Could you check a few things on this model? Use its own coordinates, in mm. Coordinates: 2 decimals unless noted, no trailing zeros. Order: outer loops, then holes, each group sorted by start corner. A loop starts at its lowest first (then second) coordinate and runs counter-clockwise, first axis right, second up. Notation, with made-up numbers: (-23, -33) -> (3, -33) arc R18 ccw to (3, -27) -> close; hole circle Ø7 at (23.25, 59.5). An arc over 180 degrees is marked (long way). Use a Markdown table: item, result. Add a question column.
1) If I drill on L1, parallel to Z at x = 15, y = 1.35; L2, parallel to Z at x = 0, y = 1.9; L3, parallel to X at y = 0.7, z = -21, over which ranges is the centre line in solid material (lowest first)? Write a range as [from, to].
2) If we section it at D-D (x = -20): Write out the boundary of the cut face in (y, z).
3) If we section it at B-B (z = 45.5): Write out the boundary of the cut face in (x, y).
4) Will these pins go through, and if not, where does the flat tip stop? pin 1 Ø0.6 at (y, z) = (1, 10.5) entering from +X; pin 2 Ø0.6 at (y, z) = (0.5, 2) entering from +X; pin 3 Ø1 at (y, z) = (0.5, -11) entering from +X; pin 4 Ø1.8 at (x, z) = (20, -34.64) entering from +Y.
5) If we section it at A-A (x = -12): Write out the boundary of the cut face in (y, z), plus the area to 3 significant figures.
6) Thinking about a two-plate mould opening in X: for faces 1 (the flat face through (28.38, 0.99, -41.2)), 2 (the flat face through (8, 2, -1)), 3 (the flat face through (-28.38, 0.99, 41.2)), 4 (the cylindrical face through (-20.45, 0.99, 33.21)), which applies, +X half, -X half, draft (parallel to the pull), parting line (faces both ways), or undercut?
7) If we section it at C-C (z = 15): Write out the boundary of the cut face in (x, y).
```python
from build123d import *

# Parameters (mm, degrees)
SKETCH1_R           = 1.5
BOSS_EXTRUDE1_DEPTH = 2
CUT_EXTRUDE1_DEPTH  = 2


with BuildPart() as part:
    # Sketch1 → Boss-Extrude1 (new body)
    with BuildSketch(Plane(origin=(0, 0, 0), x_dir=(1, 0, 0), z_dir=(0, 1, 0))):
        with BuildLine():
            Line((-31.856435644, 6.435643564), (-25, 75))
            Line((-25, 75), (25, 75))
            Line((25, 75), (31.856435644, 6.435643564))
            ThreePointArc((31.856435644, 6.435643564), (32.5, 0), (31.856435644, -6.435643564))
            Line((31.856435644, -6.435643564), (25, -75))
            Line((25, -75), (-25, -75))
            Line((-25, -75), (-31.856435644, -6.435643564))
            ThreePointArc((-31.856435644, -6.435643564), (-32.5, 0), (-31.856435644, 6.435643564))
        make_face()
        with Locations(Location((-20, 34.641016151, 0), (0, 0, 270))):
            Circle(SKETCH1_R, mode=Mode.SUBTRACT)
        with Locations(Location((20, 34.641016151, 0), (0, 0, 90))):
            Circle(SKETCH1_R, mode=Mode.SUBTRACT)
        with Locations(Location((20, -34.641016151, 0), (0, 0, 270))):
            Circle(SKETCH1_R, mode=Mode.SUBTRACT)
        with Locations(Location((-20, -34.641016151, 0), (0, 0, 90))):
            Circle(SKETCH1_R, mode=Mode.SUBTRACT)
    extrude(amount=BOSS_EXTRUDE1_DEPTH)

    # Sketch2 → Cut-Extrude1 (cut)
    with BuildSketch(Plane(origin=(0, 2, 0), x_dir=(1, 0, 0), z_dir=(0, 1, 0))):
        with BuildLine():
            Line((-15, 70), (15, 70))
            ThreePointArc((15, 70), (16.5, 68.5), (15, 67))
            Line((15, 67), (-15, 67))
            ThreePointArc((-15, 67), (-16.5, 68.5), (-15, 70))
        make_face()
        with BuildLine():
            Line((-15, -70), (15, -70))
            ThreePointArc((15, -70), (16.5, -68.5), (15, -67))
            Line((15, -67), (-15, -67))
            ThreePointArc((-15, -67), (-16.5, -68.5), (-15, -70))
        make_face()
        with BuildLine():
            Line((-15, 44), (15, 44))
            ThreePointArc((15, 44), (16.5, 45.5), (15, 47))
            Line((15, 47), (-15, 47))
            ThreePointArc((-15, 47), (-16.5, 45.5), (-15, 44))
        make_face()
        with BuildLine():
            Line((-15, -44), (15, -44))
            ThreePointArc((15, -44), (16.5, -45.5), (15, -47))
            Line((15, -47), (-15, -47))
            ThreePointArc((-15, -47), (-16.5, -45.5), (-15, -44))
        make_face()
        with BuildLine():
            Line((-18.5, 24.682455481), (-18.5, -24.682555481))
            ThreePointArc((-18.5, -24.682555481), (-20, -26.182555481), (-21.5, -24.682555481))
            Line((-21.5, -24.682555481), (-21.5, 24.682455481))
            ThreePointArc((-21.5, 24.682455481), (-20, 26.182455481), (-18.5, 24.682455481))
        make_face()
        with BuildLine():
            Line((18.5, 24.682455481), (18.5, -24.682555481))
            ThreePointArc((18.5, -24.682555481), (20, -26.182555481), (21.5, -24.682555481))
            Line((21.5, -24.682555481), (21.5, 24.682455481))
            ThreePointArc((21.5, 24.682455481), (20, 26.182455481), (18.5, 24.682455481))
        make_face()
        with BuildLine():
            Line((1.5, 25), (1.5, -25))
            ThreePointArc((1.5, -25), (0, -26.5), (-1.5, -25))
            Line((-1.5, -25), (-1.5, 25))
            ThreePointArc((-1.5, 25), (0, 26.5), (1.5, 25))
        make_face()
    extrude(amount=-CUT_EXTRUDE1_DEPTH, mode=Mode.SUBTRACT)


solid = part.part
```
Answer sheet:
| question | item | result |
|---|---|---|
| 1 | L1 | [-75, -70], [-67, -47], [-44, 44], [47, 67], [70, 75] |
| 1 | L2 | [-75, -70], [-67, -47], [-44, -26.5], [26.5, 44], [47, 67], [70, 75] |
| 1 | L3 | [-30.4, -21.5], [-18.5, -1.5], [1.5, 18.5], [21.5, 30.4] |
| 2 | outline | (0, -75) -> (2, -75) -> (2, -36.14) -> (0, -36.14) -> close; (0, -33.14) -> (2, -33.14) -> (2, -26.18) -> (0, -26.18) -> close; (0, 26.18) -> (2, 26.18) -> (2, 33.14) -> (0, 33.14) -> close; (0, 36.14) -> (2, 36.14) -> (2, 75) -> (0, 75) -> close |
| 3 | outline | (-27.95, 0) -> (-16.5, 0) -> (-16.5, 2) -> (-27.95, 2) -> close; (16.5, 0) -> (27.95, 0) -> (27.95, 2) -> (16.5, 2) -> close |
| 4 | pin 1 | x = 31.48 |
| 4 | pin 2 | x = 32.46 |
| 4 | pin 3 | x = 31.45 |
| 4 | pin 4 | through |
| 5 | outline | (0, -75) -> (2, -75) -> (2, -70) -> (0, -70) -> close; (0, -67) -> (2, -67) -> (2, -47) -> (0, -47) -> close; (0, -44) -> (2, -44) -> (2, 44) -> (0, 44) -> close; (0, 47) -> (2, 47) -> (2, 67) -> (0, 67) -> close; (0, 70) -> (2, 70) -> (2, 75) -> (0, 75) -> close |
| 5 | area | 276 mm2 |
| 6 | face 1 | +X half |
| 6 | face 2 | draft |
| 6 | face 3 | -X half |
| 6 | face 4 | undercut |
| 7 | outline | (-31, 0) -> (-21.5, 0) -> (-21.5, 2) -> (-31, 2) -> close; (-18.5, 0) -> (-1.5, 0) -> (-1.5, 2) -> (-18.5, 2) -> close; (1.5, 0) -> (18.5, 0) -> (18.5, 2) -> (1.5, 2) -> close; (21.5, 0) -> (31, 0) -> (31, 2) -> (21.5, 2) -> close |
